Input: part model. Units: mm. Frame: model coordinates. Face numbers are marked on the shaded views. A direction names the side the tool comes from. Round coordinates to 2 decimals unless told otherwise and drop trailing zeros. Write each loop counter-clockwise with the first axis right and the second up, starting at its lowest first coordinate (ties: lowest second). Pieces come first, ordered by that corner, then holes. Notation, with made-up numbers: (70.5, 75.25) -> (118.5, 75.25) arc R13 ccw to (118.5, 95.25) -> close; hole circle Ø8 at (7.25, 22). An arc over 180 degrees is marked (long way). Use CSV: the item, a comma, the result in double quotes.
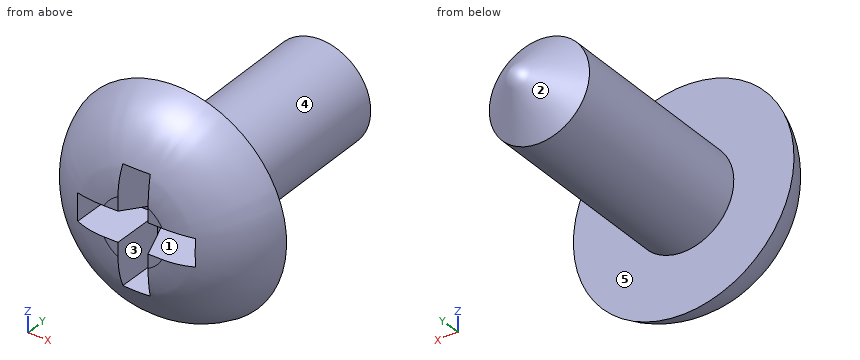
```python
from build123d import *

# Parameters (mm, degrees)
SKETCH1_R           = 1.25
BOSS_EXTRUDE1_DEPTH = 5
SKETCH2_R           = 2.75
BOSS_EXTRUDE2_DEPTH = 1.5
FILLET1_R           = 2
CUT_EXTRUDE1_DEPTH  = 1
CUT_EXTRUDE1_DRAFT  = -15


with BuildPart() as part:
    # Sketch1 → Boss-Extrude1 (new body)
    with BuildSketch(Plane(origin=(0, 0, 0), x_dir=(1, 0, 0), z_dir=(0, 1, 0))):
        with Locations(Location((0, 0, 0), (0, 0, 270))):
            Circle(SKETCH1_R)
    extrude(amount=BOSS_EXTRUDE1_DEPTH)

    # Sketch2 → Boss-Extrude2 (add)
    with BuildSketch(Plane.XZ):
        with Locations(Location((0, 0, 0), (0, 0, 270))):
            Circle(SKETCH2_R)
    extrude(amount=BOSS_EXTRUDE2_DEPTH)

    # Fillet1
    # the kernel refuses this fillet: 2 mm, written as the material it takes off along each edge
    with BuildSketch(Plane(origin=(0, -1.5, 0), x_dir=(0, 0, -1), z_dir=(-1, 0, 0))) as fillet1_piece_1:
        with BuildLine():
            CenterArc((0.813508327, -2), FILLET1_R, 14.477512186, 75.522487814)
            Line((0.813508327, 0), (0.813508327, 0.04))
            Line((0.813508327, 0.04), (2.75, 0.04))
            Line((2.75, 0.04), (2.79, 0))
            ThreePointArc((2.79, 0), (2.79, -0.75), (2.788729833, -1.49))
            Line((2.788729833, -1.49), (2.75, -1.5))
        make_face()
    revolve(axis=Axis((0, -1.5, 0), (0, -1, 0)), mode=Mode.SUBTRACT)


with BuildPart() as cut_extrude1_tool:
    # Sketch3 → Cut-Extrude1 (with draft: the straight prism first)
    with BuildSketch(Plane.XZ.offset(1.5)):
        Polygon((0.375, 0.375), (0.375, 1.5), (-0.375, 1.5), (-0.375, 0.375), (-1.5, 0.375), (-1.5, -0.375), (-0.375, -0.375), (-0.375, -1.5), (0.375, -1.5), (0.375, -0.375), (1.5, -0.375), (1.5, 0.375), align=None)
    extrude(amount=-CUT_EXTRUDE1_DEPTH)
    # Cut-Extrude1: the draft: its side faces are tilted about the plane it starts from
    cut_extrude1_sides = [cut_extrude1_tool.faces().sort_by_distance(p)[0] for p in [
        (0.375, -1, 0.9375),
        (0, -1, 1.5),
        (-0.375, -1, 0.9375),
        (-0.9375, -1, 0.375),
        (-1.5, -1, 0),
        (-0.9375, -1, -0.375),
        (-0.375, -1, -0.9375),
        (0, -1, -1.5),
        (0.375, -1, -0.9375),
        (0.9375, -1, -0.375),
        (1.5, -1, 0),
        (0.9375, -1, 0.375),
    ]]
    draft(cut_extrude1_sides, Plane.XZ.offset(1.5), CUT_EXTRUDE1_DRAFT)


with BuildPart() as part_1:
    add(part.part)

    # Cut-Extrude1: cut by cut_extrude1_tool
    add(cut_extrude1_tool.part, mode=Mode.SUBTRACT)

    # Sketch11 → Revolve2 (revolve)
    with BuildSketch(Plane.XY, mode=Mode.PRIVATE) as revolve2_sk:
        Polygon((0, 5), (0, 6), (-1.25, 5), align=None)
    revolve(revolve2_sk.sketch.rotate(Axis((0, 5, 0), (0, 1, 0)), 103.11828208), axis=Axis((0, 5, 0), (0, 1, 0)))


solid = part_1.part
```
Item 1: Section query A-A on y = 3. Return the cut outline in (x, z), plus the area to 3 significant figures.
Worked answers:
outline,"circle Ø2.5 at (0, 0)"
area,"4.91 mm²"
Item 2: Pull-direction query (Z, two-part tool) for the marked faces 3, 4 and 5; classes: +Z half, -Z half, draft (parallel to the pull), parting line (faces both ways), or undercut.
Worked answers:
face 3,"undercut"
face 4,"parting line"
face 5,"draft"
Item 3: First-contact query: pin 1 Ø1.5 at (y, z) = (2.5, 1.5) entering from -X; pin 2 Ø2 at (y, z) = (4, 0) entering from -X; pin 3 Ø1.5 at (x, y) = (1.5, 3) entering from -Z; pin 4 Ø2.5 at (x, z) = (0, -0.5) entering from -Y. Flat tips, straight axial feed; report the tip coordinate or a pass-through.
Worked answers:
pin 1,"stops at x = -1"
pin 2,"stops at x = -1.25"
pin 3,"stops at z = -1"
pin 4,"stops at y = -1.5"
Item 4: Line query: line 1 (Y direction, x = 0.95, z = -1.5); line 2 (X direction, y = 1.5, z = 0.05); line 3 (Z direction, x = 0.2, y = 2). Output: solid intervals per line, ascending.
Worked answers:
line 1,"y = -1.25 to 0"
line 2,"x = -1.25 to 1.25"
line 3,"z = -1.23 to 1.23"
Item 5: Section query B-B on y = 5.25. Return the cut outline in (x, z) (1 decimal), plus the area to 3 significant figures.
Worked answers:
outline,"circle Ø1.9 at (0, 0)"
area,"2.76 mm²"
Item 6: Set-up query: the marked faces 1 and 2. Return all of +Z, -Z, +X, -X, +Y, -Y with unobstructed straight access to the full face (end or side cutting, diameter ignored); none if empty.
Worked answers:
face 1,"-Y"
face 2,"+Y"
